```python
from build123d import *

# Parameters (mm, degrees)
SKETCH4_R           = 3.175
SKETCH4_R_2         = 1.75
BOSS_EXTRUDE1_DEPTH = 6.35


with BuildPart() as part:
    # Sketch4 → Boss-Extrude1 (new body)
    with BuildSketch(Plane.XY):
        with BuildLine():
            Line((43.977135669, 255.932866189), (75.839955751, 249.270355141))
            ThreePointArc((75.839955751, 249.270355141), (83.108950302, 253.320349798), (80.127586616, 261.089018222))
            Line((80.127586616, 261.089018222), (51.40452772, 276.406140819))
            ThreePointArc((51.40452772, 276.406140819), (35.887988835, 270.451395034), (43.977135669, 255.932866189))
        make_face()
        with Locations((46.228541785, 266.7)):
            Circle(SKETCH4_R, mode=Mode.SUBTRACT)
        with Locations((53.74894393, 263.971712703)):
            Circle(SKETCH4_R_2, mode=Mode.SUBTRACT)
        with Locations((77.139631099, 255.485927841)):
            Circle(SKETCH4_R_2, mode=Mode.SUBTRACT)
        with Locations((43.500254487, 259.179597855)):
            Circle(SKETCH4_R_2, mode=Mode.SUBTRACT)
        with Locations((38.708139639, 269.428287297)):
            Circle(SKETCH4_R_2, mode=Mode.SUBTRACT)
        with Locations((48.956829082, 274.220402145)):
            Circle(SKETCH4_R_2, mode=Mode.SUBTRACT)
    extrude(amount=BOSS_EXTRUDE1_DEPTH)


solid = part.part
```
Check sheet for the modelled part. Datum: model origin and axes. Units: mm. Round coordinates to 2 decimals unless told otherwise and drop trailing zeros. Order: outer loops, then holes, each group sorted by start corner. A loop starts at its lowest first (then second) coordinate and runs counter-clockwise, first axis right, second up. Notation, with made-up numbers: M 21.5,-5.5 L 25.5,-5.5 A14 ccw 25.5,0.5 Z; hole C 83.25,13.25 d2. An arc over 180 degrees is marked long. Answer in a Markdown table with one row per item.
(1) Draft check along X on faces 1 (the flat face through (65.97, 268.64, 3.13)), 2 (the cylindrical face through (44.31, 257.63, 3.13)), 3 (the flat face through (59, 260, 0)), 4 (the cylindrical face through (35.98, 270.7, 3.13)). Enter one of: +X half, -X half, draft (parallel to the pull), parting line (faces both ways), or undercut.
Findings:
| item | result |
|---|---|
| face 1 | +X half |
| face 2 | undercut |
| face 3 | draft |
| face 4 | parting line |
(2) Section check D-D on x = 68.5. Record the boundary of the cut face in (y, z).
Findings:
| item | result |
|---|---|
| outline | M 250.81,0 L 267.29,0 L 267.29,6.35 L 250.81,6.35 Z |
(3) Section check B-B on x = 42.5. Record the boundary of the cut face in (y, z).
Findings:
| item | result |
|---|---|
| outline | M 256.35,0 L 257.74,0 L 257.74,6.35 L 256.35,6.35 Z; M 260.62,0 L 277.05,0 L 277.05,6.35 L 260.62,6.35 Z |
(4) Gauge pin test, flat ends, axial feed: pin 1 (3 mm diameter, centred on x = 48.5, z = 4, fed in from +Y); pin 2 (2 mm diameter, centred on x = 53.5, z = 2, fed in from -Y). Record the tip position at first contact, or that the pin passes through.
Findings:
| item | result |
|---|---|
| pin 1 | stops at y = 277.67 |
| pin 2 | stops at y = 253.73 |
(5) Section check C-C on z = 0.5. Record the boundary of the cut face in (x, y) (3 decimals), plus the area to 3 significant figures.
Findings:
| item | result |
|---|---|
| outline | M 43.977,255.933 L 75.84,249.27 A6.35 ccw 80.128,261.089 L 51.405,276.406 A11 ccw long Z; hole C 38.708,269.428 d3.5; hole C 43.5,259.18 d3.5; hole C 46.229,266.7 d6.35; hole C 48.957,274.22 d3.5; hole C 53.749,263.972 d3.5; hole C 77.14,255.486 d3.5 |
| area | 750 mm^2 |
(6) Material ranges on line 1 along X through (y, z) = (268.5, 4.5); line 2 along X through (y, z) = (266.7, 4.75); line 3 along X through (y, z) = (258, 4.5), recorded low to high. Write a range as from..to.
Findings:
| item | result |
|---|---|
| line 1 | x = 35.38..37.22, 40.19..43.61, 48.84..66.23 |
| line 2 | x = 35.23..43.05, 49.4..69.61 |
| line 3 | x = 39.5..42.21, 44.79..82.97 |
(7) Section check A-A on y = 256.75. Record the boundary of the cut face in (x, z).
Findings:
| item | result |
|---|---|
| outline | M 41.54,0 L 75.93,0 L 75.93,6.35 L 41.54,6.35 Z; M 78.35,0 L 83.36,0 L 83.36,6.35 L 78.35,6.35 Z |
